The listing builds one solid part. Answer for the finished solid, in the listing's coordinates (mm). A direction names the side the tool comes from. Round coordinates to 2 decimals unless told otherwise and drop trailing zeros. Write each loop counter-clockwise with the first axis right and the second up, starting at its lowest first coordinate (ties: lowest second). Pieces come first, ordered by that corner, then holes. Notation, with made-up numbers: (32, 13) - (53, 13) arc R33 cw to (53, 47) - close; hole circle Ø11 at (72.25, 51.5). An arc over 180 degrees is marked (long way). Answer as CSV lines item,"result". Start each with the question number.
Item 1: A cutting plane is placed at D-D on x = 7.5. Determine the outline of the cut face in (y, z).
Item 2: Flat-ended cylindrical pins translate along their axes: pin 1 (0.5 mm diameter, centred on x = 7.5, y = 1, fed in from +Z); pin 2 (1.5 mm diameter, centred on y = 3, z = 2.5, fed in from -X); pin 3 (0.9 mm diameter, centred on x = 4.5, z = 1.5, fed in from +Y). Find the tip coordinate at first contact, or state that the pin passes through.
Item 3: For a pull along Y with two mould halves and no side action, classify faces 4 (the cylindrical face through (4.56, 2.25, 0.83)), 5 (the cylindrical face through (0.285, 0.301, 0.247)), 6 (the flat face through (4, 2, 0)) as pulls with the +Y half, pulls with the -Y half, needs draft (parallel to the pull), parting line crosses it, or undercut.
Item 4: Straight lines are drawn through the part: line 1 along Y through (x, z) = (6.5, 1.8); line 2 along Z through (x, y) = (2.5, 2); line 3 along Z through (x, y) = (8.5, 3.1). For each, find the intervals that lie inside material, in ascending order. Write a range as [from, to].
Item 5: Which of the six approach directions +Z, -Z, +X, -X, +Y, -Y give full straight-line access (tool end or side, diameter ignored) to faces 1 (the cylindrical face through (8.715, 3.699, 0.247)), 2 (the flat face through (4, 3.5, 2)), 3 (the flat face through (4, 0.5, 2))?
Item 6: A cutting plane is placed at C-C on z = 0.9. Determine the outline of the cut face in (x, y).
Item 7: A cutting plane is placed at B-B on x = 6.25. Determine the outline of the cut face in (y, z).
```python
from build123d import *

# Parameters (mm, degrees)
F0_W         = 5
F0_H         = 3
F1_DEPTH     = 3.25
F0_W_2       = 9
F0_H_2       = 4
F2_DEPTH     = 1
F5_DEPTH     = 12.5
F6_T1_DEPTH  = 4
F6_T3_DEPTH  = 2
F6_T5_DEPTH  = 1.75
F6_S9_W      = 0.5
F6_S9_H      = 0.5
F6_T10_DEPTH = 0.5
F6_S15_W     = 0.5
F6_S15_H     = 0.5
F6_T16_DEPTH = 0.5
F6_S21_W     = 0.5
F6_S21_H     = 0.5
F6_T22_DEPTH = 0.5
F6_S27_W     = 0.5
F6_S27_H     = 0.5
F6_T28_DEPTH = 0.5
F6_T34_ANGLE = 359.64
F7_T1_DEPTH  = 15
F7_T3_DEPTH  = 7.4
F7_T5_DEPTH  = 7.4
F8_T1_DEPTH  = 3.5
F8_T4_ANGLE  = 90
F8_T6_ANGLE  = 90
F8_T8_ANGLE  = 90
F8_T10_ANGLE = 90


# Not quite as in the source:
# - a fillet or chamfer that OpenCascade refuses, or shapes differently, is made with other operations: its cross-section is extruded or revolved along the edge and cut away or added
# - a feature names something its author has since deleted; it is built from what else it names


with BuildPart() as f1:
    # F0 (on Top) → F1 (new body)
    with BuildSketch(Plane.XY):
        with Locations((4.5, 2)):
            Rectangle(F0_W, F0_H)
    extrude(amount=F1_DEPTH)

    # F0 (on Top) → F2 (join)
    with BuildSketch(Plane.XY):
        with Locations((4.5, 2)):
            Rectangle(F0_W_2, F0_H_2)
        with Locations((4.5, 2)):
            Rectangle(F0_W, F0_H, mode=Mode.SUBTRACT)
    extrude(amount=F2_DEPTH)

    # F4 (on face) → F5 (cut, symmetric)
    with BuildSketch(Plane.YZ.offset(7)):
        with BuildLine():
            Line((2.6, 1), (1.4, 1))
            ThreePointArc((1.4, 1), (2, 0.8), (2.6, 1))
        make_face()
        with BuildLine():
            ThreePointArc((2.6, 1), (2.894427191, 1.3527864045), (3, 1.8))
            ThreePointArc((3, 1.8), (1.5527864045, 2.694427191), (1.4, 1))
            Line((1.4, 1), (2.6, 1))
        make_face()
    extrude(amount=F5_DEPTH, both=True, mode=Mode.SUBTRACT)

    # F6: fillet of radius 0.5 on 9 edges, made by hand

    # F6_s2 → F6_t1 (cut)
    with BuildSketch(Plane.YZ.offset(2.5)):
        with BuildLine():
            ThreePointArc((0.5, 2.75), (0.6464466094, 3.1035533906), (1, 3.25))
            Line((1, 3.25), (0.5, 3.25))
            Line((0.5, 3.25), (0.5, 2.75))
        make_face()
        with BuildLine():
            ThreePointArc((3, 3.25), (3.3535533906, 3.1035533906), (3.5, 2.75))
            Line((3.5, 2.75), (3.5, 3.25))
            Line((3.5, 3.25), (3, 3.25))
        make_face()
    extrude(amount=F6_T1_DEPTH, mode=Mode.SUBTRACT)

    # F6_s4 → F6_t3 (cut)
    with BuildSketch(Plane.XZ.offset(-3)):
        with BuildLine():
            ThreePointArc((6.5, 3.25), (6.8535533906, 3.1035533906), (7, 2.75))
            Line((7, 2.75), (7, 3.25))
            Line((7, 3.25), (6.5, 3.25))
        make_face()
        with BuildLine():
            ThreePointArc((2, 2.75), (2.1464466094, 3.1035533906), (2.5, 3.25))
            Line((2.5, 3.25), (2, 3.25))
            Line((2, 3.25), (2, 2.75))
        make_face()
    extrude(amount=F6_T3_DEPTH, mode=Mode.SUBTRACT)

    # F6_s6 → F6_t5 (cut)
    with BuildSketch(Plane.XY.offset(1)):
        with BuildLine():
            ThreePointArc((6.5, 0.5), (6.8535533906, 0.6464466094), (7, 1))
            Line((7, 1), (7, 0.5))
            Line((7, 0.5), (6.5, 0.5))
        make_face()
        with BuildLine():
            ThreePointArc((6.5, 3.5), (6.8535533906, 3.3535533906), (7, 3))
            Line((7, 3), (7, 3.5))
            Line((7, 3.5), (6.5, 3.5))
        make_face()
        with BuildLine():
            ThreePointArc((2, 1), (2.1464466094, 0.6464466094), (2.5, 0.5))
            Line((2.5, 0.5), (2, 0.5))
            Line((2, 0.5), (2, 1))
        make_face()
        with BuildLine():
            ThreePointArc((2, 3), (2.1464466094, 3.3535533906), (2.5, 3.5))
            Line((2.5, 3.5), (2, 3.5))
            Line((2, 3.5), (2, 3))
        make_face()
    extrude(amount=F6_T5_DEPTH, mode=Mode.SUBTRACT)


with BuildPart() as f6_tool8:
    # F6_s9 → F6_t10 (new body)
    with BuildSketch(Plane.YZ.offset(2.5)):
        with Locations((0.75, 3)):
            Rectangle(F6_S9_W, F6_S9_H)
    extrude(amount=-F6_T10_DEPTH)

    # F6_s11 → F6_t12 (revolve, cut)
    with BuildSketch(Plane(origin=(2.5, 1, 2.75), x_dir=(0, 0.7071067812, -0.7071067812), z_dir=(0, 0.7071067812, 0.7071067812))):
        with BuildLine():
            ThreePointArc((0, -0.5), (0.5, 0), (0, 0.5))
            Line((0, 0.5), (0, -0.5))
        make_face()
    revolve(axis=Axis((2.5, 1, 2.75), (-1, 0, 0)), mode=Mode.SUBTRACT)


with BuildPart() as f1_1:
    add(f1.part)

    # F6_t7: cut F6_tool8
    add(f6_tool8.part, mode=Mode.SUBTRACT)


with BuildPart() as f6_tool14:
    # F6_s15 → F6_t16 (new body)
    with BuildSketch(Plane.YZ.offset(6.5)):
        with Locations((0.75, 3)):
            Rectangle(F6_S15_W, F6_S15_H)
    extrude(amount=F6_T16_DEPTH)

    # F6_s17 → F6_t18 (revolve, cut)
    with BuildSketch(Plane(origin=(6.5, 1, 2.75), x_dir=(0, 0.7071067812, -0.7071067812), z_dir=(0, -0.7071067812, -0.7071067812))):
        with BuildLine():
            ThreePointArc((0, -0.5), (0.5, 0), (0, 0.5))
            Line((0, 0.5), (0, -0.5))
        make_face()
    revolve(axis=Axis((6.5, 1, 2.75), (1, 0, 0)), mode=Mode.SUBTRACT)


with BuildPart() as f1_2:
    add(f1_1.part)

    # F6_t13: cut F6_tool14
    add(f6_tool14.part, mode=Mode.SUBTRACT)


with BuildPart() as f6_tool20:
    # F6_s21 → F6_t22 (new body)
    with BuildSketch(Plane.YZ.offset(6.5)):
        with Locations((3.25, 3)):
            Rectangle(F6_S21_W, F6_S21_H)
    extrude(amount=F6_T22_DEPTH)

    # F6_s23 → F6_t24 (revolve, cut)
    with BuildSketch(Plane(origin=(6.5, 3, 2.75), x_dir=(0, -0.7071067812, -0.7071067812), z_dir=(0, -0.7071067812, 0.7071067812))):
        with BuildLine():
            ThreePointArc((0, -0.5), (0.5, 0), (0, 0.5))
            Line((0, 0.5), (0, -0.5))
        make_face()
    revolve(axis=Axis((6.5, 3, 2.75), (1, 0, 0)), mode=Mode.SUBTRACT)


with BuildPart() as f1_3:
    add(f1_2.part)

    # F6_t19: cut F6_tool20
    add(f6_tool20.part, mode=Mode.SUBTRACT)


with BuildPart() as f6_tool26:
    # F6_s27 → F6_t28 (new body)
    with BuildSketch(Plane.YZ.offset(2.5)):
        with Locations((3.25, 3)):
            Rectangle(F6_S27_W, F6_S27_H)
    extrude(amount=-F6_T28_DEPTH)

    # F6_s29 → F6_t30 (revolve, cut)
    with BuildSketch(Plane(origin=(2.5, 3, 2.75), x_dir=(0, -0.7071067812, -0.7071067812), z_dir=(0, 0.7071067812, -0.7071067812))):
        with BuildLine():
            ThreePointArc((0, -0.5), (0.5, 0), (0, 0.5))
            Line((0, 0.5), (0, -0.5))
        make_face()
    revolve(axis=Axis((2.5, 3, 2.75), (-1, 0, 0)), mode=Mode.SUBTRACT)


with BuildPart() as f1_4:
    add(f1_3.part)

    # F6_t25: cut F6_tool26
    add(f6_tool26.part, mode=Mode.SUBTRACT)


with BuildPart() as f6_tool32:
    # F6_s33 → F6_t34 (revolve)
    with BuildSketch(Plane(origin=(0, 2.0056350904, 0.0063009092), x_dir=(1, 0, 0), z_dir=(0, -0.9999950652, -0.0031415875))):
        with BuildLine():
            ThreePointArc((6.5, 0.7937079424), (6.8535533906, 0.647261333), (7, 0.2937079424))
            Line((7, 0.2937079424), (7, 0.7937079424))
            Line((7, 0.7937079424), (6.5, 0.7937079424))
        make_face()
    revolve(axis=Axis((7, 2, 1.8), (1, 0, 0)), revolution_arc=F6_T34_ANGLE)

    split(bisect_by=Plane.XY.offset(1), keep=Keep.TOP)


with BuildPart() as f1_5:
    add(f1_4.part)

    # F6_t31: cut F6_tool32
    add(f6_tool32.part, mode=Mode.SUBTRACT)

    # F7: fillet of radius 0.5 on 4 edges, made by hand

    # F7_s2 → F7_t1 (cut)
    with BuildSketch(Plane.YZ.offset(-3)):
        with BuildLine():
            ThreePointArc((3.5, 1), (3.8535533906, 0.8535533906), (4, 0.5))
            Line((4, 0.5), (4.01, 0.5))
            Line((4.01, 0.5), (4.01, 1.01))
            Line((4.01, 1.01), (3.5, 1.01))
            Line((3.5, 1.01), (3.5, 1))
        make_face()
        with BuildLine():
            ThreePointArc((0.5, 1), (0.1464466094, 0.8535533906), (0, 0.5))
            Line((0, 0.5), (-0.01, 0.5))
            Line((-0.01, 0.5), (-0.01, 1.01))
            Line((-0.01, 1.01), (0.5, 1.01))
            Line((0.5, 1.01), (0.5, 1))
        make_face()
    extrude(amount=F7_T1_DEPTH, mode=Mode.SUBTRACT)

    # F7_s4 → F7_t3 (cut)
    with BuildSketch(Plane.XZ.offset(-4.4)):
        with BuildLine():
            ThreePointArc((0.5, 1), (0.1464466094, 0.8535533906), (0, 0.5))
            Line((0, 0.5), (-0.01, 0.5))
            Line((-0.01, 0.5), (-0.01, 1.01))
            Line((-0.01, 1.01), (0.5, 1.01))
            Line((0.5, 1.01), (0.5, 1))
        make_face()
    extrude(amount=F7_T3_DEPTH, mode=Mode.SUBTRACT)

    # F7_s6 → F7_t5 (cut)
    with BuildSketch(Plane.XZ.offset(-7)):
        with BuildLine():
            ThreePointArc((8.5, 1), (8.8535533906, 0.8535533906), (9, 0.5))
            Line((9, 0.5), (9.01, 0.5))
            Line((9.01, 0.5), (9.01, 1.01))
            Line((9.01, 1.01), (8.5, 1.01))
            Line((8.5, 1.01), (8.5, 1))
        make_face()
    extrude(amount=F7_T5_DEPTH, mode=Mode.SUBTRACT)

    # F8: fillet of radius 1 on 4 edges, made by hand

    # F8_s2 → F8_t1 (cut)
    with BuildSketch(Plane.XY.offset(-2.5)):
        with BuildLine():
            ThreePointArc((9, 1), (8.7071067812, 0.2928932188), (8, 0))
            Line((8, 0), (9, 0))
            Line((9, 0), (9, 1))
        make_face()
        with BuildLine():
            ThreePointArc((9, 3), (8.7071067812, 3.7071067812), (8, 4))
            Line((8, 4), (9, 4))
            Line((9, 4), (9, 3))
        make_face()
        with BuildLine():
            ThreePointArc((0, 1), (0.2928932188, 0.2928932188), (1, 0))
            Line((1, 0), (0, 0))
            Line((0, 0), (0, 1))
        make_face()
        with BuildLine():
            ThreePointArc((0, 3), (0.2928932188, 3.7071067812), (1, 4))
            Line((1, 4), (0, 4))
            Line((0, 4), (0, 3))
        make_face()
    extrude(amount=F8_T1_DEPTH, mode=Mode.SUBTRACT)

    # F8_s3 → F8_t4 (revolve, cut)
    with BuildSketch(Plane.YZ.offset(1)):
        with BuildLine():
            ThreePointArc((3.5, 1), (3.8535533906, 0.8535533906), (4, 0.5))
            Line((4, 0.5), (4, 1))
            Line((4, 1), (3.5, 1))
        make_face()
    revolve(axis=Axis((1, 3, 1), (0, 0, 1)), revolution_arc=F8_T4_ANGLE, mode=Mode.SUBTRACT)

    # F8_s5 → F8_t6 (revolve, cut)
    with BuildSketch(Plane.XZ.offset(-1)):
        with BuildLine():
            ThreePointArc((0.5, 1), (0.1464466094, 0.8535533906), (0, 0.5))
            Line((0, 0.5), (0, 1))
            Line((0, 1), (0.5, 1))
        make_face()
    revolve(axis=Axis((1, 1, 1), (0, 0, 1)), revolution_arc=F8_T6_ANGLE, mode=Mode.SUBTRACT)

    # F8_s7 → F8_t8 (revolve, cut)
    with BuildSketch(Plane.XZ.offset(-3)):
        with BuildLine():
            ThreePointArc((8.5, 1), (8.8535533906, 0.8535533906), (9, 0.5))
            Line((9, 0.5), (9, 1))
            Line((9, 1), (8.5, 1))
        make_face()
    revolve(axis=Axis((8, 3, 1), (0, 0, 1)), revolution_arc=F8_T8_ANGLE, mode=Mode.SUBTRACT)

    # F8_s9 → F8_t10 (revolve, cut)
    with BuildSketch(Plane.YZ.offset(8)):
        with BuildLine():
            ThreePointArc((0.5, 1), (0.1464466094, 0.8535533906), (0, 0.5))
            Line((0, 0.5), (0, 1))
            Line((0, 1), (0.5, 1))
        make_face()
    revolve(axis=Axis((8, 1, 1), (0, 0, 1)), revolution_arc=F8_T10_ANGLE, mode=Mode.SUBTRACT)


solid = f1_5.part
```
Geometry says:
1,outline,"(0, 0) - (4, 0) - (4, 0.5) arc R0.5 ccw to (3.5, 1) - (2.6, 1) arc R1 cw to (1.4, 1) - (0.5, 1) arc R0.5 ccw to (0, 0.5) - close"
2,pin 1,"stops at z = 1"
2,pin 2,"stops at x = 2"
2,pin 3,"stops at y = 3.5"
3,face 4,"undercut"
3,face 5,"pulls with the -Y half"
3,face 6,"needs draft"
4,line 1,"y = [0.5, 1], [3, 3.5]"
4,line 2,"z = [0, 0.8], [2.8, 3.25]"
4,line 3,"z = [0, 1]"
5,face 1,"+Z, -Z, +X, +Y"
5,face 2,"+Z, +X, -X, +Y"
5,face 3,"+Z, +X, -X, -Y"
6,outline,"(0.2, 1) arc R0.8 ccw to (1, 0.2) - (8, 0.2) arc R0.8 ccw to (8.8, 1) - (8.8, 1.56) - (0.2, 1.56) - close; (0.2, 2.44) - (8.8, 2.44) - (8.8, 3) arc R0.8 ccw to (8, 3.8) - (1, 3.8) arc R0.8 ccw to (0.2, 3) - close"
7,outline,"(0, 0) - (4, 0) - (4, 0.5) arc R0.5 ccw to (3.5, 1) - (3.5, 2.75) arc R0.5 ccw to (3, 3.25) - (1, 3.25) arc R0.5 ccw to (0.5, 2.75) - (0.5, 1) arc R0.5 ccw to (0, 0.5) - close; hole circle Ø2 at (2, 1.8)"
